Work out the finished part from the listing and answer in its coordinate system (mm). Face numbers are marked on the shaded views. Round coordinates to 2 decimals unless told otherwise and drop trailing zeros. Order: outer loops, then holes, each group sorted by start corner. A loop starts at its lowest first (then second) coordinate and runs counter-clockwise, first axis right, second up. Notation, with made-up numbers: (-8, -27) - (26, -27) arc R11 ccw to (26, -14) - close; hole circle Ø4 at (-5, 83). An arc over 180 degrees is marked (long way). Use one line per item in the form item = value. Start each with the question number.
Q1. For a pull along X with two mould halves and no side action, classify the marked faces 1, 2 and 3 as +X half, -X half, draft (parallel to the pull), parting line (faces both ways), or undercut.
Q2. The part is cut by section A-A on z = -13.3. Determine the outline of the cut face in (x, y).
Q3. The part is cut by section B-B on x = -33. Determine the outline of the cut face in (y, z).
Q4. Find the intervals of material crossed by line 1 (Z direction, x = -1, y = 1); line 2 (X direction, y = 0.75, z = -5.5); line 3 (Y direction, x = -23.5, z = -32), in increasing order. Write a range as [from, to].
Q5. Given P1, Ø0.7, axis at x = 12, y = 1.5, coming from the +Z side; P2, Ø12, axis at x = -10, z = -27.5, coming from the -Y side; P3, Ø6, axis at x = -31.75, z = -13.3, coming from the +Y side; P4, Ø2.5, axis at x = -10.5, y = 1, coming from the -Z side, each flat-ended and moving along its own axis, determine where each tip first touches the part or whether it passes through.
Q6. The part is cut by section D-D on z = -20.5. Determine the outline of the cut face in (x, y).
Q7. The part is cut by section C-C on y = -1.75. Determine the outline of the cut face in (x, z).
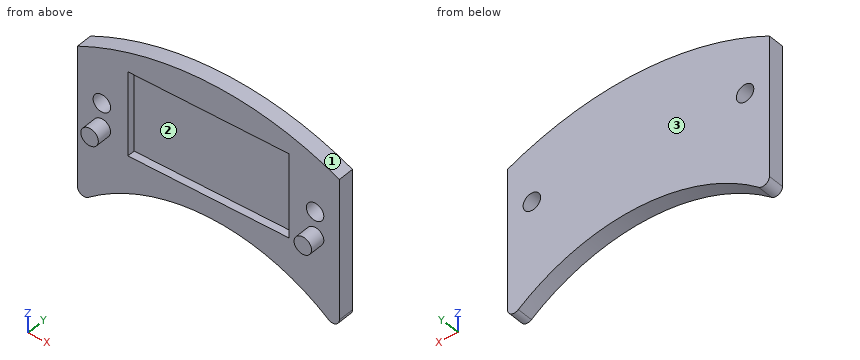
from build123d import *

# Parameters (mm, degrees)
F1_DEPTH = 4.8
F2_R     = 2.6
F3_DEPTH = 4.5
F4_R     = 2.6
F5_DEPTH = 4.8
F6_R     = 2
F7_W     = 48
F7_H     = 2.3
F8_DEPTH = 25


with BuildPart() as f1:
    # F0 (on Front) → F1 (new body)
    with BuildSketch(Plane.XZ):
        with BuildLine():
            Line((-39, 0), (-39, -46))
            ThreePointArc((-39, -46), (0, -31), (39, -46))
            Line((39, -46), (39, 0))
            ThreePointArc((39, 0), (0, 9), (-39, 0))
        make_face()
    extrude(amount=-F1_DEPTH)

    # F2 (on face) → F3 (join)
    with BuildSketch(Plane.XZ):
        with Locations((-31.75, -20.5)):
            Circle(F2_R)
        with Locations((31.75, -20.5)):
            Circle(F2_R)
    extrude(amount=F3_DEPTH)

    # F4 (on face) → F5 (cut, through all)
    with BuildSketch(Plane(origin=(0, 4.8, 0), x_dir=(-1, 0, 0), z_dir=(0, 1, 0))):
        with Locations((-31.75, -13.3)):
            Circle(F4_R)
        with Locations((31.75, -13.3)):
            Circle(F4_R)
    extrude(amount=-F5_DEPTH, mode=Mode.SUBTRACT)

    # F6
    f6_edges = [f1.edges().sort_by_distance(p)[0] for p in [
        (-39, 2.4, -46),
        (39, 2.4, -46),
    ]]
    fillet(f6_edges, radius=F6_R)

    # F7 (on Top) → F8 (cut)
    with BuildSketch(Plane.XY):
        with Locations((0, 1.15)):
            Rectangle(F7_W, F7_H)
    extrude(amount=-F8_DEPTH, mode=Mode.SUBTRACT)


solid = f1.part
Found:
q1.face_1 = parting line
q1.face_2 = undercut
q1.face_3 = draft
q2.outline = (-39, 0) - (-34.35, 0) - (-34.35, 4.8) - (-39, 4.8) - close; (-29.15, 0) - (-24, 0) - (-24, 2.3) - (24, 2.3) - (24, 0) - (29.15, 0) - (29.15, 4.8) - (-29.15, 4.8) - close; (34.35, 0) - (39, 0) - (39, 4.8) - (34.35, 4.8) - close
q3.outline = (-4.5, -22.78) - (0, -22.78) - (0, -41.26) - (4.8, -41.26) - (4.8, -15.58) - (0, -15.58) - (0, -18.22) - (-4.5, -18.22) - close; (0, -11.02) - (4.8, -11.02) - (4.8, 2.66) - (0, 2.66) - close
q4.line_1 = [-31.01, -25], [0, 8.99]
q4.line_2 = [-39, -24], [24, 39]
q4.line_3 = [0, 4.8]
q5.P1 = 8.23
q5.P2 = 0
q5.P3 = 4.8
q5.P4 = -32.2
q6.outline = (-39, 0) - (-34.35, 0) - (-34.35, -4.5) - (-29.15, -4.5) - (-29.15, 0) - (-24, 0) - (-24, 2.3) - (24, 2.3) - (24, 0) - (29.15, 0) - (29.15, -4.5) - (34.35, -4.5) - (34.35, 0) - (39, 0) - (39, 4.8) - (-39, 4.8) - close
q7.outline = circle Ø5.2 at (-31.75, -20.5); circle Ø5.2 at (31.75, -20.5)
